Input: part model. Units: mm. Frame: model coordinates. A direction names the side the tool comes from. Give positions to 0.01 mm unless a question says otherwise; leave off trailing zeros. Loops run counter-clockwise (first coordinate to the right, second up) from the corner with the lowest first, then second, coordinate; pieces in that order, holes last. Notation, with made-up numbers: (55.25, 10.5) - (112.25, 10.5) arc R12 ccw to (112.25, 14.5) - close; hole circle Ø10 at (89.25, -18.5). An arc over 180 degrees is marked (long way). Answer as a JSON object with one key per item and string values.
from build123d import *

# Parameters (mm, degrees)
PAD_DEPTH       = 14.7
POCKET_DEPTH    = 11.7
SKETCH012_R     = 10
SKETCH012_R_2   = 4
PAD003_DEPTH    = 7
SKETCH015_R     = 1
SKETCH015_W     = 8
SKETCH015_H     = 4
POCKET003_DEPTH = 6
POCKET004_DEPTH = 4.1
SKETCH013_R     = 3.75
POCKET001_DEPTH = 3
POCKET002_DEPTH = 1.6
SKETCH017_R     = 2
POCKET005_DEPTH = 5.2
FILLET_R        = 1


with BuildPart() as part:
    # Sketch → Pad (new body)
    with BuildSketch(Plane.XY):
        with BuildLine():
            Line((-162, 6), (162, 6))
            ThreePointArc((166, 2), (164.828427, 4.828427), (162, 6))
            Line((166, 2), (166, -232))
            ThreePointArc((162, -236), (164.828427, -234.828427), (166, -232))
            Line((162, -236), (-162, -236))
            ThreePointArc((-166, -232), (-164.828427, -234.828427), (-162, -236))
            Line((-166, -232), (-166, 2))
            ThreePointArc((-162, 6), (-164.828427, 4.828427), (-166, 2))
        make_face()
    extrude(amount=PAD_DEPTH)

    # Sketch001 → Pocket (cut)
    with BuildSketch(Plane.XY.offset(14.7)):
        with BuildLine():
            Line((-137.593576, 0.5), (138.406481, 0.5))
            ThreePointArc((141.406424, -2.518402), (140.534297, -0.385196), (138.406481, 0.5))
            Line((141.406424, -2.518402), (140.49521, -151.068141))
            ThreePointArc((137.495267, -154.049739), (139.610071, -153.177555), (140.49521, -151.068141))
            Line((137.495267, -154.049739), (-137.593576, -154.049739))
            ThreePointArc((-140.593576, -151.049739), (-139.714896, -153.171059), (-137.593576, -154.049739))
            Line((-140.593576, -151.049739), (-140.593576, -2.5))
            ThreePointArc((-137.593576, 0.5), (-139.714896, -0.37868), (-140.593576, -2.5))
        make_face()
    extrude(amount=-POCKET_DEPTH, mode=Mode.SUBTRACT)

    # Sketch012 → Pad003 (join)
    with BuildSketch(Plane.XY):
        with Locations((-70, -120)):
            Circle(SKETCH012_R)
        with Locations((70, -120)):
            Circle(SKETCH012_R)
        with Locations((70, -30)):
            Circle(SKETCH012_R)
        with Locations((0, -90)):
            Circle(SKETCH012_R)
        with Locations((-70, -30)):
            Circle(SKETCH012_R)
        with Locations((40, -10)):
            Circle(SKETCH012_R_2)
        with Locations((-40, -10)):
            Circle(SKETCH012_R_2)
    extrude(amount=PAD003_DEPTH)

    # Sketch015 → Pocket003 (cut)
    with BuildSketch(Plane.XZ):
        with Locations((-11.3, 5.25)):
            Circle(SKETCH015_R)
        with BuildLine():
            ThreePointArc((2.75, 3), (5, 5.25), (2.75, 7.5))
            Line((2.75, 7.5), (-2.75, 7.5))
            ThreePointArc((-2.75, 7.5), (-5, 5.25), (-2.75, 3))
            Line((-2.75, 3), (2.75, 3))
        make_face()
        with Locations((24.384758, 5)):
            Rectangle(SKETCH015_W, SKETCH015_H)
    extrude(amount=-POCKET003_DEPTH, mode=Mode.SUBTRACT)

    # Sketch016 → Pocket004 (cut)
    with BuildSketch(Plane.XZ.offset(-1.9)):
        with BuildLine():
            Line((-4, 9.425651), (28, 9.425651))
            ThreePointArc((31, 6.425651), (30.12132, 8.546971), (28, 9.425651))
            Line((31, 6.425651), (31, 4.425651))
            ThreePointArc((28, 1.425651), (30.12132, 2.304331), (31, 4.425651))
            Line((28, 1.425651), (-4, 1.425651))
            ThreePointArc((-7, 4.425651), (-6.12132, 2.304331), (-4, 1.425651))
            Line((-7, 4.425651), (-7, 6.425651))
            ThreePointArc((-4, 9.425651), (-6.12132, 8.546971), (-7, 6.425651))
        make_face()
    extrude(amount=-POCKET004_DEPTH, mode=Mode.SUBTRACT)

    # Sketch013 → Pocket001 (cut)
    with BuildSketch(Plane.XY.offset(7)):
        with Locations((-70, -30)):
            Circle(SKETCH013_R)
        with Locations((-70, -120)):
            Circle(SKETCH013_R)
        with Locations((70, -120)):
            Circle(SKETCH013_R)
        with Locations((70, -30)):
            Circle(SKETCH013_R)
        with Locations((0, -90)):
            Circle(SKETCH013_R)
    extrude(amount=-POCKET001_DEPTH, mode=Mode.SUBTRACT)

    # Sketch014 → Pocket002 (cut)
    with BuildSketch(Plane.XY.offset(14.7)):
        with BuildLine():
            Line((-157, 0.5), (157, 0.5))
            ThreePointArc((161, -3.5), (159.828427, -0.671573), (157, 0.5))
            Line((161, -3.5), (161, -226.5))
            ThreePointArc((157, -230.5), (159.828427, -229.328427), (161, -226.5))
            Line((157, -230.5), (-157, -230.5))
            ThreePointArc((-161, -226.5), (-159.828427, -229.328427), (-157, -230.5))
            Line((-161, -226.5), (-161, -3.5))
            ThreePointArc((-157, 0.5), (-159.828427, -0.671573), (-161, -3.5))
        make_face()
    extrude(amount=-POCKET002_DEPTH, mode=Mode.SUBTRACT)

    # Sketch017 → Pocket005 (cut)
    with BuildSketch(Plane.XY.offset(13.1)):
        with Locations((-150, -10)):
            Circle(SKETCH017_R)
        with Locations((-150, -220)):
            Circle(SKETCH017_R)
        with Locations((150, -10)):
            Circle(SKETCH017_R)
        with Locations((150, -220)):
            Circle(SKETCH017_R)
    extrude(amount=-POCKET005_DEPTH, mode=Mode.SUBTRACT)

    # Fillet
    fillet_edges = [part.edges().sort_by_distance(p)[0] for p in [
        (-166, -115, 14.7),
        (-164.828427, -234.828427, 14.7),
        (0, -236, 14.7),
        (0, 6, 14.7),
        (-164.828427, 4.828427, 14.7),
        (164.828427, 4.828427, 14.7),
        (166, -115, 14.7),
        (164.828427, -234.828427, 14.7),
    ]]
    fillet(fillet_edges, radius=FILLET_R)


solid = part.part
Item 1: Cut plane A-A (x = 89.5). Return loops of the section in (y, z), then the cut area to 3 significant figures.
Geometry check:
{"outline": "(-236, 0) - (6, 0) - (6, 13.7) arc R1 ccw to (5, 14.7) - (0.5, 14.7) - (0.5, 3) - (-154.05, 3) - (-154.05, 13.1) - (-230.5, 13.1) - (-230.5, 14.7) - (-235, 14.7) arc R1 ccw to (-236, 13.7) - close", "area": "1,630 mm2"}
Item 2: Contact query for flat-ended pins moving along their axis: P1, Ø6, axis at x = -63.5, y = -29, coming from the +Z side; P2, Ø12, axis at x = -30.5, y = -114, coming from the +Z side; P3, Ø10, axis at x = -70, y = -30, coming from the -Z side; P4, Ø6.5, axis at x = 6.5, z = 6, coming from the +Y side. Output: stop coordinate, or through.
Geometry check:
{"P1": "stops at z = 7", "P2": "stops at z = 3", "P3": "stops at z = 0", "P4": "stops at y = 1.9"}
Item 3: Cut plane C-C (x = -40). Return loops of the section in (y, z).
Geometry check:
{"outline": "(-236, 0) - (6, 0) - (6, 13.7) arc R1 ccw to (5, 14.7) - (0.5, 14.7) - (0.5, 3) - (-6, 3) - (-6, 7) - (-14, 7) - (-14, 3) - (-154.05, 3) - (-154.05, 13.1) - (-230.5, 13.1) - (-230.5, 14.7) - (-235, 14.7) arc R1 ccw to (-236, 13.7) - close"}
Item 4: Mould query, pull axis Y, two halves, no side actions, for faces 1 (the face through (73.577, -28.874, 5.521)), 2 (the face through (-70, -34, 7)), 3 (the face through (-2, -113, 0)), 4 (the face through (-2, 6, 10)). Classes: released by +Y, released by -Y, zero draft, split by the parting line, or undercut.
Geometry check:
{"face 1": "undercut", "face 2": "undercut", "face 3": "zero draft", "face 4": "released by +Y"}
Item 5: Cut plane D-D (y = -145). Return loops of the section in (x, z).
Geometry check:
{"outline": "(-166, 0) - (166, 0) - (166, 13.7) arc R1 ccw to (165, 14.7) - (161, 14.7) - (161, 13.1) - (140.53, 13.1) - (140.53, 3) - (-140.59, 3) - (-140.59, 13.1) - (-161, 13.1) - (-161, 14.7) - (-165, 14.7) arc R1 ccw to (-166, 13.7) - close"}
Item 6: Access query for faces 5 (the face through (12, 1.9, 5)), 6 (the face through (-80, -30, 5)), 7 (the face through (1, 1, 14.7)). Directions: +Z, -Z, +X, -X, +Y, -Y. A direction counts if a zero-diameter tool reaches every point of the face in a straight line with its end or side. Return the directions, or none.
Geometry check:
{"face 5": "+Y", "face 6": "+Z", "face 7": "+Z, +X, -X, +Y, -Y"}
Item 7: Material intervals for line 1 (Y direction, x = 0, z = 5.95); line 2 (Y direction, x = 70, z = 5.4); line 3 (Y direction, x = -150, z = 9.35), sorted ascending. Write a range as [from, to].
Geometry check:
{"line 1": "y = [-236, -154.05], [-100, -93.75], [-86.25, -80]", "line 2": "y = [-236, -154.05], [-130, -123.75], [-116.25, -110], [-40, -33.75], [-26.25, -20], [0.5, 6]", "line 3": "y = [-236, -222], [-218, -12], [-8, 6]"}
